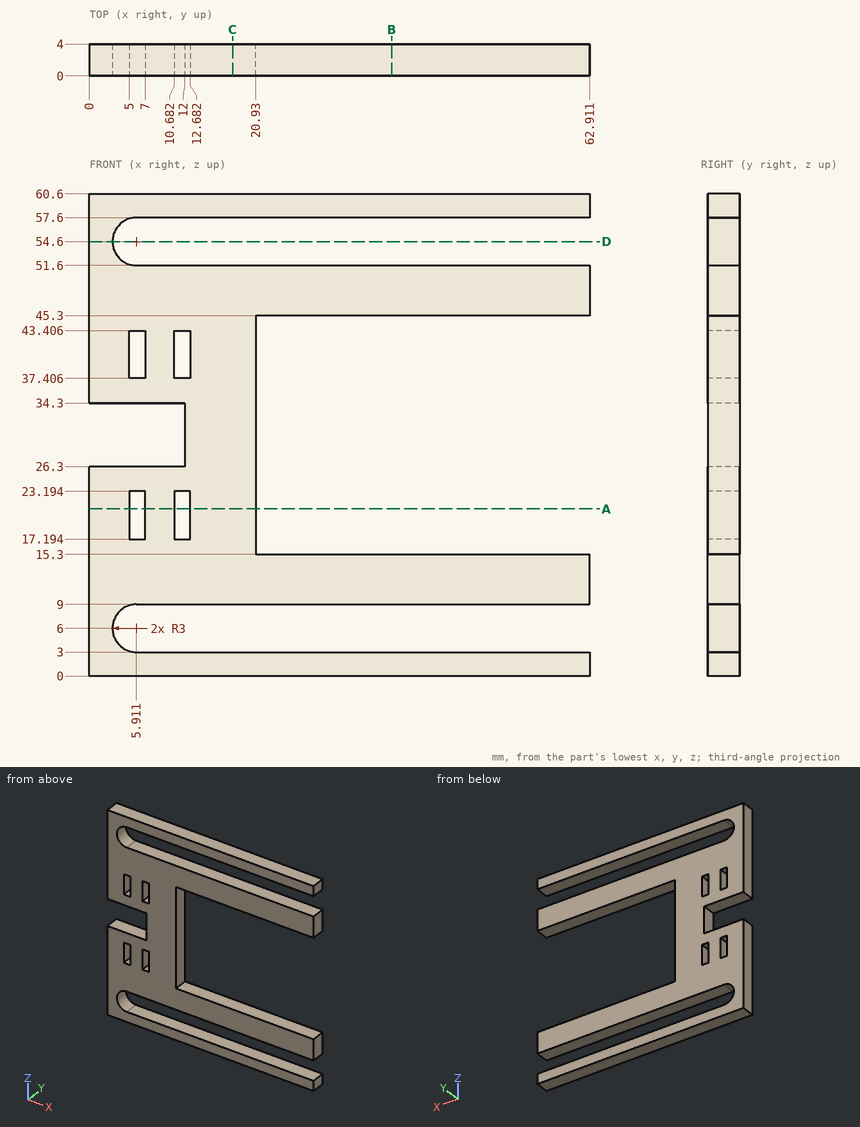
Verification items for this drawing (mm, ordinates from the low corner). Round coordinates to 2 decimals unless told otherwise and drop trailing zeros. Order: outer loops, then holes, each group sorted by start corner. A loop starts at its lowest first (then second) coordinate and runs counter-clockwise, first axis right, second up. Notation, with made-up numbers: (-32, -36.75) - (0, -36.75) arc R10 cw to (0, -27.75) - close; hole circle Ø6 at (53.25, -17). An arc over 180 degrees is marked (long way). Answer as CSV lines item,"result". Start each with the question number.
1) Section check D-D (z = 54.6). Record the cut outline in (x, y), then the cut area to 3 significant figures.
2) Scan lines: probe 1 along Z at (x, y) = (49.5, 1.75); probe 2 along Z at (x, y) = (8, 0.9); probe 3 along X at (y, z) = (2.35, 21). Record each from-to range of solid material in increasing order.
3) Section check A-A (z = 21). Record the cut outline in (x, y).
4) Section check C-C (x = 18). Record the cut outline in (y, z), then the cut area to 3 significant figures.
5) Section check B-B (x = 38). Record the cut outline in (y, z), then the cut area to 3 significant figures.
6) Depth check by flat-ended pin: pin 1 (2 mm diameter, centred on y = 2, z = 29.5, fed in from -X); pin 2 (1.2 mm diameter, centred on y = 2.5, z = 20.5, fed in from +X). Enter the tip coordinate at first touch or a pass-through.
Determined:
1,outline,"(0, 0) - (2.91, 0) - (2.91, 4) - (0, 4) - close"
1,area,"11.6 mm^2"
2,probe 1,"0 to 3, 9 to 15.3, 45.3 to 51.6, 57.6 to 60.6"
2,probe 2,"0 to 3, 9 to 26.3, 34.3 to 51.6, 57.6 to 60.6"
2,probe 3,"0 to 5, 7 to 10.68, 12.68 to 20.93"
3,outline,"(0, 0) - (5, 0) - (5, 4) - (0, 4) - close; (7, 0) - (10.68, 0) - (10.68, 4) - (7, 4) - close; (12.68, 0) - (20.93, 0) - (20.93, 4) - (12.68, 4) - close"
4,outline,"(0, 0) - (4, 0) - (4, 3) - (0, 3) - close; (0, 9) - (4, 9) - (4, 51.6) - (0, 51.6) - close; (0, 57.6) - (4, 57.6) - (4, 60.6) - (0, 60.6) - close"
4,area,"194 mm^2"
5,outline,"(0, 0) - (4, 0) - (4, 3) - (0, 3) - close; (0, 9) - (4, 9) - (4, 15.3) - (0, 15.3) - close; (0, 45.3) - (4, 45.3) - (4, 51.6) - (0, 51.6) - close; (0, 57.6) - (4, 57.6) - (4, 60.6) - (0, 60.6) - close"
5,area,"74.4 mm^2"
6,pin 1,"x = 12"
6,pin 2,"x = 20.93"
